from build123d import *

# Parameters (mm, degrees)
SKETCH1_W                                     = 45
SKETCH1_H                                     = 105
BOSS_EXTRUDE1_DEPTH                           = 10
FILLET1_R                                     = 5
CUT_EXTRUDE1_DEPTH                            = 10
CSK_FOR_M5_COUNTERSUNK_FLAT_HEAD1_D           = 5.5
CSK_FOR_M5_COUNTERSUNK_FLAT_HEAD1_DEPTH       = 30
CSK_FOR_M5_COUNTERSUNK_FLAT_HEAD1_CSINK_D     = 10.4
CSK_FOR_M5_COUNTERSUNK_FLAT_HEAD1_CSINK_ANGLE = 90
CSK_FOR_M5_COUNTERSUNK_FLAT_HEAD1_TIP         = 1.652366702


with BuildPart() as part:
    # Sketch1 → Boss-Extrude1 (new body)
    with BuildSketch(Plane.XY):
        with Locations((22.5, 52.5)):
            Rectangle(SKETCH1_W, SKETCH1_H)
    extrude(amount=BOSS_EXTRUDE1_DEPTH)

    # Fillet1
    fillet1_edges = [part.edges().sort_by_distance(p)[0] for p in [
        (0, 105, 5),
        (45, 105, 5),
        (45, 0, 5),
        (0, 0, 5),
    ]]
    fillet(fillet1_edges, radius=FILLET1_R)

    # Sketch2 → Cut-Extrude1 (cut)
    with BuildSketch(Plane.XY.offset(10)):
        with BuildLine():
            Line((12.5, 20), (12.5, 8))
            ThreePointArc((12.5, 8), (8.75, 4.25), (5, 8))
            Line((5, 8), (5, 20))
            ThreePointArc((5, 20), (8.75, 23.75), (12.5, 20))
        make_face()
        with BuildLine():
            Line((12.5, 72), (12.5, 62))
            ThreePointArc((12.5, 62), (8.75, 58.25), (5, 62))
            Line((5, 62), (5, 72))
            ThreePointArc((5, 72), (8.75, 75.75), (12.5, 72))
        make_face()
        with BuildLine():
            Line((32.5, 20), (32.5, 8))
            ThreePointArc((32.5, 8), (36.25, 4.25), (40, 8))
            Line((40, 8), (40, 20))
            ThreePointArc((40, 20), (36.25, 23.75), (32.5, 20))
        make_face()
        with BuildLine():
            Line((32.5, 72), (32.5, 62))
            ThreePointArc((32.5, 62), (36.25, 58.25), (40, 62))
            Line((40, 62), (40, 72))
            ThreePointArc((40, 72), (36.25, 75.75), (32.5, 72))
        make_face()
        with BuildLine():
            Line((32.5, 85), (32.5, 97))
            ThreePointArc((32.5, 97), (36.25, 100.75), (40, 97))
            Line((40, 97), (40, 85))
            ThreePointArc((40, 85), (36.25, 81.25), (32.5, 85))
        make_face()
        with BuildLine():
            Line((32.5, 33), (32.5, 43))
            ThreePointArc((32.5, 43), (36.25, 46.75), (40, 43))
            Line((40, 43), (40, 33))
            ThreePointArc((40, 33), (36.25, 29.25), (32.5, 33))
        make_face()
        with BuildLine():
            Line((12.5, 85), (12.5, 97))
            ThreePointArc((12.5, 97), (8.75, 100.75), (5, 97))
            Line((5, 97), (5, 85))
            ThreePointArc((5, 85), (8.75, 81.25), (12.5, 85))
        make_face()
        with BuildLine():
            Line((26.25, 85), (26.25, 97))
            ThreePointArc((26.25, 97), (22.5, 100.75), (18.75, 97))
            Line((18.75, 97), (18.75, 85))
            ThreePointArc((18.75, 85), (22.5, 81.25), (26.25, 85))
        make_face()
        with BuildLine():
            Line((26.25, 20), (26.25, 8))
            ThreePointArc((26.25, 8), (22.5, 4.25), (18.75, 8))
            Line((18.75, 8), (18.75, 20))
            ThreePointArc((18.75, 20), (22.5, 23.75), (26.25, 20))
        make_face()
        with BuildLine():
            Line((12.5, 33), (12.5, 43))
            ThreePointArc((12.5, 43), (8.75, 46.75), (5, 43))
            Line((5, 43), (5, 33))
            ThreePointArc((5, 33), (8.75, 29.25), (12.5, 33))
        make_face()
    extrude(amount=-CUT_EXTRUDE1_DEPTH, mode=Mode.SUBTRACT)

    # CSK for M5 Countersunk Flat Head1
    with Locations(Plane.XY.offset(10)):
        with Locations((22.5, 60.5), (22.5, 44.5)):
            CounterSinkHole(CSK_FOR_M5_COUNTERSUNK_FLAT_HEAD1_D / 2, CSK_FOR_M5_COUNTERSUNK_FLAT_HEAD1_CSINK_D / 2, depth=CSK_FOR_M5_COUNTERSUNK_FLAT_HEAD1_DEPTH, counter_sink_angle=CSK_FOR_M5_COUNTERSUNK_FLAT_HEAD1_CSINK_ANGLE)
            with Locations((0, 0, -(CSK_FOR_M5_COUNTERSUNK_FLAT_HEAD1_DEPTH + CSK_FOR_M5_COUNTERSUNK_FLAT_HEAD1_TIP / 2))):  # 118° drill point
                Cone(0, CSK_FOR_M5_COUNTERSUNK_FLAT_HEAD1_D / 2, CSK_FOR_M5_COUNTERSUNK_FLAT_HEAD1_TIP, mode=Mode.SUBTRACT)


solid = part.part
Geometry: final body of the model. Coordinates: model frame, mm. A direction names the side the tool comes from. Coordinates: 2 decimals unless noted, no trailing zeros. Write each loop counter-clockwise with the first axis right and the second up, starting at its lowest first coordinate (ties: lowest second). Pieces come first, ordered by that corner, then holes. Notation, with made-up numbers: (-31.5, 13) - (14.5, 13) arc R28 ccw to (14.5, 49) - close; hole circle Ø1 at (37, 87). An arc over 180 degrees is marked (long way). Return JSON: item names as keys, results as strings.
Item 1: Section query D-D (x = 6). Output: boundary loops of the cut face in (y, z), and give its area (3 significant figures).
Completed:
{"outline": "(0, 0) - (5.45, 0) - (5.45, 10) - (0, 10) - close; (22.55, 0) - (30.45, 0) - (30.45, 10) - (22.55, 10) - close; (45.55, 0) - (59.45, 0) - (59.45, 10) - (45.55, 10) - close; (74.55, 0) - (82.45, 0) - (82.45, 10) - (74.55, 10) - close; (99.55, 0) - (105, 0) - (105, 10) - (99.55, 10) - close", "area": "406 mm2"}
Item 2: Section query C-C (z = 4). Count the separate pieces of the cut face and the enclosed holes in it, and give its area (3 significant figures).
Completed:
{"separate pieces": "1", "enclosed holes": "12", "area": "3,370 mm2"}
Item 3: Pin query (flat end, axial travel): pin 1 Ø3 at (x, y) = (14, 34) entering from -Z; pin 2 Ø9 at (x, y) = (22.5, 60.5) entering from +Z. Return the tip coordinate at first contact, or that it passes through.
Completed:
{"pin 1": "stops at z = 0", "pin 2": "stops at z = 9.3"}
Item 4: Pull-direction query (Y, two-part tool) for faces 3 (the face through (5, 38, 5)), 4 (the face through (44, 103, 5)), 5 (the face through (22, 0, 5)); classes: +Y half, -Y half, draft (parallel to the pull), parting line (faces both ways), or undercut.
Completed:
{"face 3": "undercut", "face 4": "+Y half", "face 5": "-Y half"}
Item 5: Section query A-A (y = 37). Output: boundary loops of the cut face in (x, z).
Completed:
{"outline": "(0, 0) - (5, 0) - (5, 10) - (0, 10) - close; (12.5, 0) - (32.5, 0) - (32.5, 10) - (12.5, 10) - close; (40, 0) - (45, 0) - (45, 10) - (40, 10) - close"}
Item 6: Reachability of faces 1 (the face through (23.12, 57.7, 7.67)), 2 (the face through (22.58, 4.25, 5.07)) from +Z, -Z, +X, -X, +Y, -Y: full face, straight path, thin tool, end or side. Return the list, or none.
Completed:
{"face 1": "+Z", "face 2": "+Z, -Z"}
Item 7: Line query: L1, parallel to X at y = 17.5, z = 8.5; L2, parallel to Y at x = 22.5, z = 4.75; L3, parallel to X at y = 69.5, z = 2.75. Output: solid intervals per line, ascending.
Completed:
{"L1": "x = 0 to 5, 12.5 to 18.75, 26.25 to 32.5, 40 to 45", "L2": "y = 0 to 4.25, 23.75 to 41.75, 47.25 to 57.75, 63.25 to 81.25, 100.75 to 105", "L3": "x = 0 to 5, 12.5 to 32.5, 40 to 45"}
Item 8: Section query B-B (x = 36.25). Output: boundary loops of the cut face in (y, z), and give its area (3 significant figures).
Completed:
{"outline": "(0, 0) - (4.25, 0) - (4.25, 10) - (0, 10) - close; (23.75, 0) - (29.25, 0) - (29.25, 10) - (23.75, 10) - close; (46.75, 0) - (58.25, 0) - (58.25, 10) - (46.75, 10) - close; (75.75, 0) - (81.25, 0) - (81.25, 10) - (75.75, 10) - close; (100.75, 0) - (105, 0) - (105, 10) - (100.75, 10) - close", "area": "310 mm2"}
